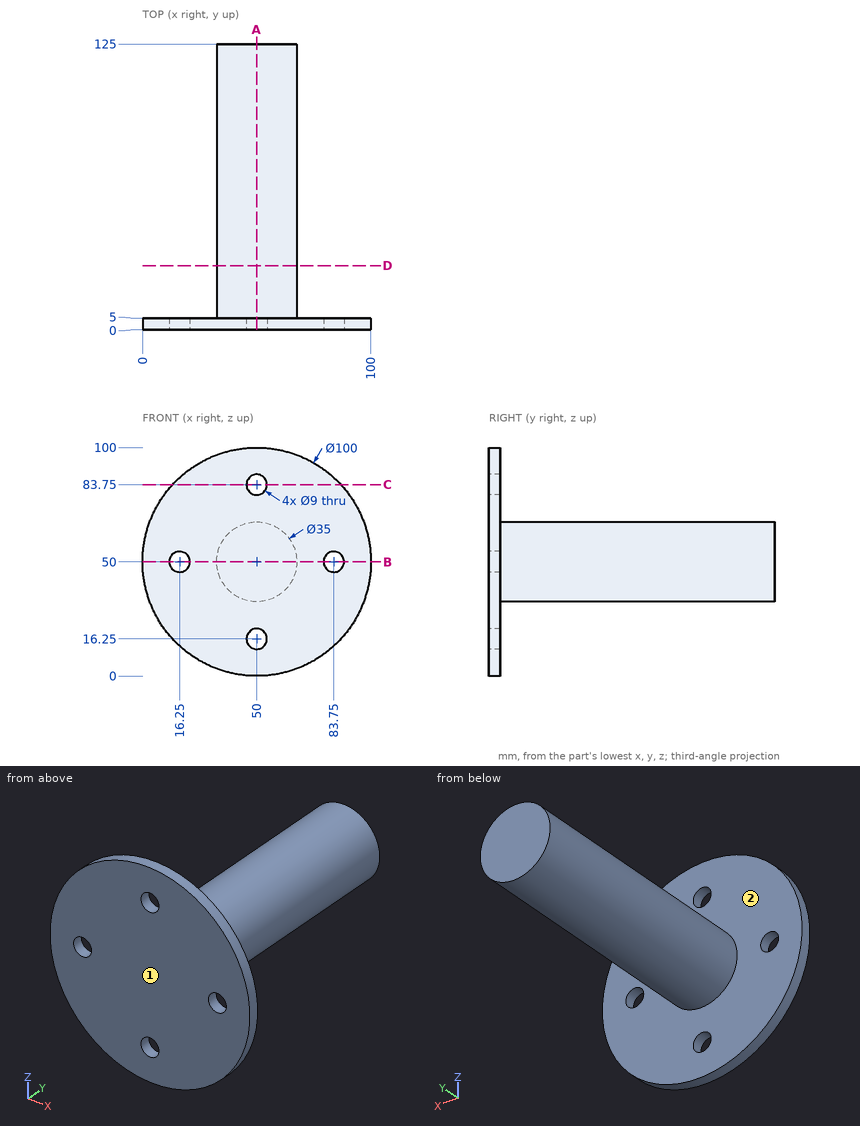
Part print with two shaded views. Sizes in mm from the minimum x, y, z corner. A direction names the side the tool comes from. Round coordinates to 2 decimals unless told otherwise and drop trailing zeros. Order: outer loops, then holes, each group sorted by start corner. A loop starts at its lowest first (then second) coordinate and runs counter-clockwise, first axis right, second up. Notation, with made-up numbers: (80.5, 2.5) -> (109.5, 2.5) arc R35 cw to (109.5, 36.5) -> close; hole circle Ø3 at (64, 28). An arc over 180 degrees is marked (long way). One line per question, with ' | ' between items.
Q1. Drop flat-ended pins along their axis: pin 1 (12 mm diameter, centred on y = 21.5, z = 39.5, fed in from -X); pin 2 (8 mm diameter, centred on y = 64, z = 43, fed in from +X); pin 3 (1.5 mm diameter, centred on x = 58.5, y = 64, fed in from -Z). Give the stop position or say it passes through.
Completed:
pin 1: stops at x = 33.09 | pin 2: stops at x = 67.24 | pin 3: stops at z = 34.31
Q2. Slice it at A-A (x = 50). Write the cut outline in (y, z).
Completed:
outline: (0, 0) -> (5, 0) -> (5, 11.75) -> (0, 11.75) -> close; (0, 20.75) -> (5, 20.75) -> (5, 32.5) -> (125, 32.5) -> (125, 67.5) -> (5, 67.5) -> (5, 79.25) -> (0, 79.25) -> close; (0, 88.25) -> (5, 88.25) -> (5, 100) -> (0, 100) -> close
Q3. Which spindle directions (+Z, -Z, +X, -X, +Y, -Y) get a long thin tool onto all of the face, cutting with end or side? Do the marked faces 1 and 2. Say none if no direction does.
Completed:
face 1: +Z, -Z, +X, -X, -Y | face 2: +Y
Q4. Slice it at C-C (z = 83.75). Write the cut outline in (x, y).
Completed:
outline: (13.11, 0) -> (45.5, 0) -> (45.5, 5) -> (13.11, 5) -> close; (54.5, 0) -> (86.89, 0) -> (86.89, 5) -> (54.5, 5) -> close
Q5. Probe probe 1 along X at (y, z) = (3.85, 50); probe 2 along Y at (x, z) = (68.5, 87.5); probe 3 along Z at (x, y) = (83, 3). List the from-to ranges inside material, lowest first.
Completed:
probe 1: x = 0 to 11.75, 20.75 to 79.25, 88.25 to 100 | probe 2: y = 0 to 5 | probe 3: z = 12.44 to 45.56, 54.44 to 87.56
Q6. Slice it at B-B (z = 50). Write the cut outline in (x, y).
Completed:
outline: (0, 0) -> (11.75, 0) -> (11.75, 5) -> (0, 5) -> close; (20.75, 0) -> (79.25, 0) -> (79.25, 5) -> (67.5, 5) -> (67.5, 125) -> (32.5, 125) -> (32.5, 5) -> (20.75, 5) -> close; (88.25, 0) -> (100, 0) -> (100, 5) -> (88.25, 5) -> close
Q7. Slice it at D-D (y = 28). Write the cut outline in (x, z), then the cut area to 3 significant figures.
Completed:
outline: circle Ø35 at (50, 50) | area: 962 mm^2
